from build123d import *

# Parameters (mm, degrees)
SKETCH1_W           = 140
SKETCH1_H           = 140
BOSS_EXTRUDE1_DEPTH = 3
CUT_EXTRUDE1_DEPTH  = 10
SKETCH3_W           = 3
SKETCH3_H           = 10
CUT_EXTRUDE2_DEPTH  = 13
SKETCH4_W           = 10
SKETCH4_H           = 3
CUT_EXTRUDE3_DEPTH  = 13


with BuildPart() as part:
    # Sketch1 → Boss-Extrude1 (new body)
    with BuildSketch(Plane(origin=(0, 0, 0), x_dir=(1, 0, 0), z_dir=(0, 1, 0))):
        Rectangle(SKETCH1_W, SKETCH1_H)
    extrude(amount=BOSS_EXTRUDE1_DEPTH)

    # Sketch2 → Cut-Extrude1 (cut)
    with BuildSketch(Plane(origin=(0, 3, 0), x_dir=(1, 0, 0), z_dir=(0, 1, 0))):
        Polygon((62, -62), (27, -62), (62, -44.9293594), align=None)
        Polygon((27, -56.436990298), (62, -39.366349698), (27, -22.295709098), align=None)
        Polygon((27, -16.732699396), (62, 0.337941204), (62, -33.803339995), align=None)
        Polygon((62, 5.900950907), (27, -11.169689693), (27, 22.971591506), align=None)
        Polygon((27, 28.534601209), (62, 45.605241809), (62, 11.463960609), align=None)
        Polygon((27, 34.097610911), (62, 51.168251511), (27, 51.168251511), align=None)
        Polygon((-27, -62), (-62, -44.9293594), (-62, -62), align=None)
        Polygon((-62, -39.366349698), (-27, -22.295709098), (-27, -56.436990298), align=None)
        Polygon((-27, -16.732699396), (-62, -33.803339995), (-62, 0.337941204), align=None)
        Polygon((-27, 22.971591506), (-62, 5.900950907), (-27, -11.169689693), align=None)
        Polygon((-27, 28.534601209), (-62, 11.463960609), (-62, 45.605241809), align=None)
        Polygon((-62, 51.168251511), (-27, 51.168251511), (-27, 34.097610911), align=None)
    extrude(amount=-CUT_EXTRUDE1_DEPTH, mode=Mode.SUBTRACT)

    # Sketch3 → Cut-Extrude2 (cut)
    with BuildSketch(Plane(origin=(0, 3, 0), x_dir=(1, 0, 0), z_dir=(0, 1, 0))):
        with Locations((68.5, -45)):
            Rectangle(SKETCH3_W, SKETCH3_H)
        with Locations((68.5, -15)):
            Rectangle(SKETCH3_W, SKETCH3_H)
        with Locations((68.5, 15)):
            Rectangle(SKETCH3_W, SKETCH3_H)
        with Locations((68.5, 45)):
            Rectangle(SKETCH3_W, SKETCH3_H)
        with Locations((-68.5, -45)):
            Rectangle(SKETCH3_W, SKETCH3_H)
        with Locations((-68.5, -15)):
            Rectangle(SKETCH3_W, SKETCH3_H)
        with Locations((-68.5, 15)):
            Rectangle(SKETCH3_W, SKETCH3_H)
        with Locations((-68.5, 45)):
            Rectangle(SKETCH3_W, SKETCH3_H)
    extrude(amount=-CUT_EXTRUDE2_DEPTH, mode=Mode.SUBTRACT)

    # Sketch4 → Cut-Extrude3 (cut)
    with BuildSketch(Plane(origin=(0, 3, 0), x_dir=(1, 0, 0), z_dir=(0, 1, 0))):
        with Locations((-45, -68.5)):
            Rectangle(SKETCH4_W, SKETCH4_H)
        with Locations((-15, -68.5)):
            Rectangle(SKETCH4_W, SKETCH4_H)
        with Locations((15, -68.5)):
            Rectangle(SKETCH4_W, SKETCH4_H)
        with Locations((45, -68.5)):
            Rectangle(SKETCH4_W, SKETCH4_H)
    extrude(amount=-CUT_EXTRUDE3_DEPTH, mode=Mode.SUBTRACT)


solid = part.part
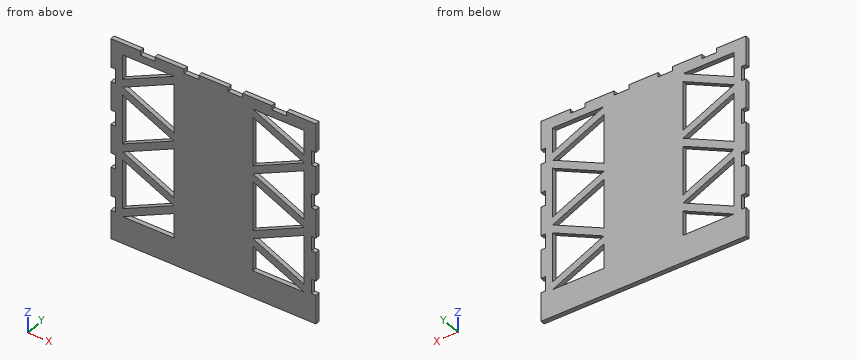
The listing builds one solid part. Answer for the finished solid, in the listing's coordinates (mm). Give positions to 0.01 mm unless a question says otherwise; leave off trailing zeros. Write each loop counter-clockwise with the first axis right and the second up, starting at its lowest first coordinate (ties: lowest second). Pieces come first, ordered by that corner, then holes.
Item 1: Section B-B, the plane z = 43 is taken. Write down the section's boundary in (x, y), plus the area to 3 significant figures.
Item 2: Flat-ended cylindrical pins translate along their axes: P1, Ø0.9, axis at y = 2, z = 46.5, coming from the -X side; P2, Ø1.5, axis at y = 1, z = 13.5, coming from the +X side; P3, Ø1, axis at x = 8.5, z = 19.5, coming from the -Y side. Find the tip coordinate at first contact, or state that the pin passes through.
Item 3: Section C-C, the plane y = 2.35 is taken. Count the separate pieces of the cut face and the enclosed holes in it, plus the area to 3 significant figures.
Item 4: Section A-A, the plane x = -43 is taken. Write down the section's boundary in (y, z).
Item 5: Find the intervals of material crossed by line 1 along X through (y, z) = (2.5, 43.5); line 2 along X through (y, z) = (2.4, -28); line 3 along X through (y, z) = (2.65, -41), in increasing order.
Item 6: Section D-D, the plane z = 8 is taken. Write down the section's boundary in (x, y).
Completed:
1. outline: (-67, 0) - (-54.55, 0) - (-54.55, 3) - (-67, 3) - close; (-27, 0) - (27, 0) - (27, 3) - (-27, 3) - close; (54.55, 0) - (67, 0) - (67, 3) - (54.55, 3) - close
1. area: 237 mm2
2. P1: stops at x = -67
2. P2: stops at x = 67
2. P3: stops at y = 0
3. separate pieces: 1
3. enclosed holes: 12
3. area: 13,300 mm2
4. outline: (0, -70) - (3, -70) - (3, -51.17) - (0, -51.17) - close; (0, -41.9) - (3, -41.9) - (3, -36.34) - (0, -36.34) - close; (0, -20.73) - (3, -20.73) - (3, -15.17) - (0, -15.17) - close; (0, 3.37) - (3, 3.37) - (3, 8.93) - (0, 8.93) - close; (0, 24.54) - (3, 24.54) - (3, 30.1) - (0, 30.1) - close; (0, 48.63) - (3, 48.63) - (3, 54.2) - (0, 54.2) - close; (0, 62) - (3, 62) - (3, 67) - (0, 67) - close
5. line 1: x = -67 to -53.52, -27 to 27, 53.52 to 67
5. line 2: x = -70 to -62, -28.1 to 28.1, 62 to 70
5. line 3: x = -67 to -62, -52.56 to -41.15, -27 to 27, 41.15 to 52.56, 62 to 67
6. outline: (-70, 0) - (-62, 0) - (-62, 3) - (-70, 3) - close; (-44.9, 0) - (-33.5, 0) - (-33.5, 3) - (-44.9, 3) - close; (-27, 0) - (27, 0) - (27, 3) - (-27, 3) - close; (33.5, 0) - (44.9, 0) - (44.9, 3) - (33.5, 3) - close; (62, 0) - (70, 0) - (70, 3) - (62, 3) - close
